Design review of the part built by this model. Coordinates are the model's own, in mm. Face numbers are marked on the shaded views. A direction names the side the tool comes from. Round coordinates to 2 decimals unless told otherwise and drop trailing zeros. Order: outer loops, then holes, each group sorted by start corner. A loop starts at its lowest first (then second) coordinate and runs counter-clockwise, first axis right, second up.
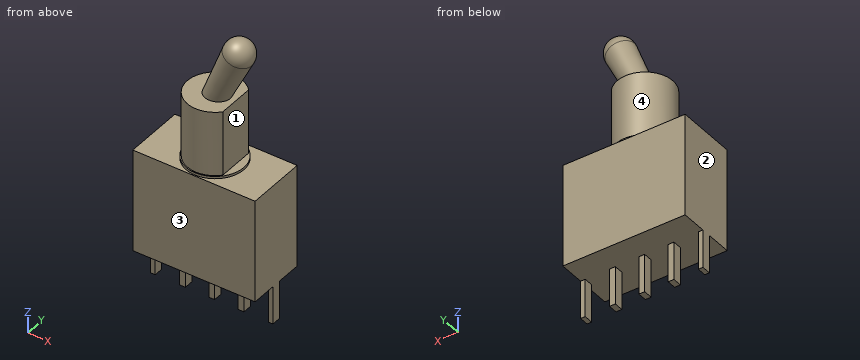
from build123d import *

# Parameters (mm, degrees)
SKETCH_W      = 10.6
SKETCH_H      = 5.2
PAD_DEPTH     = 8.9
SKETCH001_R   = 2.5
PAD001_DEPTH  = 0.2
SKETCH002_R   = 2.4
PAD002_DEPTH  = 5.6
SKETCH003_W   = 0.5
SKETCH003_H   = 0.8
SKETCH003_W_2 = 0.4
PAD003_DEPTH  = 3.3
SKETCH004_W   = 5.3
SKETCH004_H   = 3.175016
POCKET_DEPTH  = 5.6


with BuildPart() as part:
    # Sketch → Pad (new body)
    with BuildSketch(Plane.XY):
        Rectangle(SKETCH_W, SKETCH_H)
    extrude(amount=PAD_DEPTH)

    # Sketch001 (on Face6 of Pad) → Pad001 (join)
    with BuildSketch(Plane.XY.offset(8.9)):
        Circle(SKETCH001_R)
    extrude(amount=PAD001_DEPTH)

    # Sketch002 (on Face8 of Pad001) → Pad002 (join)
    with BuildSketch(Plane.XY.offset(9.1)):
        Circle(SKETCH002_R)
    extrude(amount=PAD002_DEPTH)

    # Sketch003 (on Face4 of Pad002) → Pad003 (join)
    with BuildSketch(Plane(origin=(0, 0, 0), x_dir=(1, 0, 0), z_dir=(0, 0, -1))):
        Rectangle(SKETCH003_W, SKETCH003_H)
        with Locations((-2.54, 0)):
            Rectangle(SKETCH003_W, SKETCH003_H)
        with Locations((2.54, 0)):
            Rectangle(SKETCH003_W, SKETCH003_H)
        with Locations((-5.1, 0)):
            Rectangle(SKETCH003_W_2, SKETCH003_H)
        with Locations((5.1, 0)):
            Rectangle(SKETCH003_W_2, SKETCH003_H)
    extrude(amount=PAD003_DEPTH)

    # Cone → Cone (revolve)
    with BuildSketch(Plane(origin=(0, 0, 14.3), x_dir=(0.9135454576, 0, -0.4067366431), z_dir=(0, -1, 0))):
        Polygon((0, 0), (1, 0), (1.25, 5.15), (0, 5.15), align=None)
    revolve(axis=Axis((0, 0, 14.3), (0.4067366431, 0, 0.9135454576)))

    # Sphere → Sphere (revolve)
    with BuildSketch(Plane(origin=(2.0946937118, 0, 19.0047591069), x_dir=(0.9135454576, 0, -0.4067366431), z_dir=(0, -1, 0))):
        with BuildLine():
            ThreePointArc((0, -1.25), (1.25, 0), (0, 1.25))
            Line((0, 1.25), (0, -1.25))
        make_face()
    revolve(axis=Axis((2.0946937118, 0, 19.0047591069), (0.4067366431, 0, 0.9135454576)))

    # Sketch004 (on Face35 of Sphere) → Pocket (cut)
    with BuildSketch(Plane(origin=(2.0946937118, 0, 14.7), x_dir=(1, 0, 0), z_dir=(0, 0, 1))):
        with Locations((2.35, 0.005894)):
            Rectangle(SKETCH004_W, SKETCH004_H)
    extrude(amount=-POCKET_DEPTH, mode=Mode.SUBTRACT)


solid = part.part
1) To check wall thickness, follow line 1 along Z through (x, y) = (-3.25, 0.45); line 2 along X through (y, z) = (-0.05, 9.25); line 3 along Z through (x, y) = (-1.5, -1.6). State the ranges of each line that lie inside material, in increasing order.
Results:
line 1: z = 0 to 8.9
line 2: x = -2.4 to 1.79
line 3: z = 0 to 14.7
2) The part is to be moulded in two halves that separate along Z. For the marked faces 1 and 2, say which applies: released by +Z, released by -Z, zero draft, split by the parting line, or undercut.
Results:
face 1: undercut
face 2: zero draft
3) For the marked faces 3 and 4, list the 3-axis set-ups (+Z, -Z, +X, -X, +Y, -Y) from which the entire face can be reached by the end or side of a thin tool; tool diameter is ignored.
Results:
face 3: +Z, -Z, +X, -X, -Y
face 4: +Z
4) Clearance check with flat-ended pins moving along their axes: P1, Ø2.5, axis at y = -0.5, z = 11.5, coming from the +X side; P2, Ø1.5, axis at x = 0.5, y = -0.5, coming from the +Z side; P3, Ø0.6, axis at x = 0, z = -2, coming from the +Y side. State where each tip first meets the part, or that it passes through.
Results:
P1: stops at x = 1.81
P2: stops at z = 19.85
P3: stops at y = 0.4
5) Take a section at C-C on x = -4. Give the boundary of the cut face in (y, z), plus the area to 3 significant figures.
Results:
outline: (-2.6, 0) - (2.6, 0) - (2.6, 8.9) - (-2.6, 8.9) - close
area: 46.3 mm2
6) Take a section at B-B on y = 2.1. Give the boundary of the cut face in (x, z), plus the area to 3 significant figures.
Results:
outline: (-5.3, 0) - (5.3, 0) - (5.3, 8.9) - (1.36, 8.9) - (1.36, 9.1) - (1.16, 9.1) - (1.16, 14.7) - (-1.16, 14.7) - (-1.16, 9.1) - (-1.36, 9.1) - (-1.36, 8.9) - (-5.3, 8.9) - close
area: 108 mm2
